For this review, take the finished solid that the model builds, in its own axes (mm). A direction names the side the tool comes from. Give positions to 0.01 mm unless a question says otherwise; leave off trailing zeros. Loops run counter-clockwise (first coordinate to the right, second up) from the corner with the lowest first, then second, coordinate; pieces in that order, holes last.
```python
from build123d import *

# Parameters (mm, degrees)
SKETCH1_R           = 6.35
BOSS_EXTRUDE1_DEPTH = 2.032
SKETCH2_R           = 4.699
BOSS_EXTRUDE2_DEPTH = 8.8646
SKETCH4_W           = 0.9906
SKETCH4_H           = 0.8509
SKETCH8_R           = 2.413
CUT_EXTRUDE2_DEPTH  = 15.24


with BuildPart() as part:
    # Sketch1 → Boss-Extrude1 (new body)
    with BuildSketch(Plane.XY):
        Circle(SKETCH1_R)
    extrude(amount=BOSS_EXTRUDE1_DEPTH)

    # Sketch2 → Boss-Extrude2 (add)
    with BuildSketch(Plane(origin=(0, 0, 0), x_dir=(-1, 0, 0), z_dir=(0, 0, -1))):
        Circle(SKETCH2_R)
    extrude(amount=BOSS_EXTRUDE2_DEPTH)

    # Sketch4 → Cut-Revolve1 (revolve, cut)
    with BuildSketch(Plane(origin=(0, 0, 0), x_dir=(0, 0, -1), z_dir=(1, 0, 0)), mode=Mode.PRIVATE) as cut_revolve1_sk:
        with Locations((7.6073, 4.27355)):
            Rectangle(SKETCH4_W, SKETCH4_H)
    revolve(cut_revolve1_sk.sketch.rotate(Axis((0, 0, 6.549062663), (0, 0, -1)), 90), axis=Axis((0, 0, 6.549062663), (0, 0, -1)), mode=Mode.SUBTRACT)

    # Sketch8 → Cut-Extrude2 (cut)
    with BuildSketch(Plane.XY.offset(2.032)):
        Circle(SKETCH8_R)
    extrude(amount=-CUT_EXTRUDE2_DEPTH, mode=Mode.SUBTRACT)


solid = part.part
```
Item 1: Tool access review of faces 5 (the cylindrical face through (-1.915, -1.468, -3.34)), 6 (the flat face through (4, 0, -7.112)), 7 (the cylindrical face through (0.61, 4.66, -3.51)): name each direction out of +Z, -Z, +X, -X, +Y, -Y from which nothing blocks a thin tool from reaching the whole face with its end or side.
Answer:
face 5: +Z, -Z
face 6: none
face 7: -Z
Item 2: Take a section at D-D on y = 0. Give the boundary of the cut face in (x, z).
Answer:
outline: (-6.35, 0) - (-4.7, 0) - (-4.7, -7.11) - (-3.85, -7.11) - (-3.85, -8.1) - (-4.7, -8.1) - (-4.7, -8.86) - (-2.41, -8.86) - (-2.41, 2.03) - (-6.35, 2.03) - close; (2.41, -8.86) - (4.7, -8.86) - (4.7, -8.1) - (3.85, -8.1) - (3.85, -7.11) - (4.7, -7.11) - (4.7, 0) - (6.35, 0) - (6.35, 2.03) - (2.41, 2.03) - close
Item 3: Take a section at C-C on z = -6.25. Give the boundary of the cut face in (x, y).
Answer:
outline: circle Ø9.4 at (0, 0); hole circle Ø4.83 at (0, 0)
Item 4: Take a section at B-B on x = 1. Give the boundary of the cut face in (y, z).
Answer:
outline: (-6.27, 0) - (-4.59, 0) - (-4.59, -7.11) - (-3.72, -7.11) - (-3.72, -8.1) - (-4.59, -8.1) - (-4.59, -8.86) - (-2.2, -8.86) - (-2.2, 2.03) - (-6.27, 2.03) - close; (2.2, -8.86) - (4.59, -8.86) - (4.59, -8.1) - (3.72, -8.1) - (3.72, -7.11) - (4.59, -7.11) - (4.59, 0) - (6.27, 0) - (6.27, 2.03) - (2.2, 2.03) - close
Item 5: Clearance check with flat-ended pins moving along their axes: pin 1 Ø6.5 at (x, y) = (1, -2) entering from -Z; pin 2 Ø1.5 at (y, z) = (-5, -5) entering from +X; pin 3 Ø2 at (y, z) = (-0.5, -3) entering from +X; pin 4 Ø1.5 at (x, z) = (-3, -4.5) entering from -Y. State where each tip first meets the part, or that it passes through.
Answer:
pin 1: stops at z = -8.86
pin 2: stops at x = 2
pin 3: stops at x = 4.7
pin 4: stops at y = -4.13
Item 6: The part is to be moulded in two halves that separate along Z. For faces 1 (the cylindrical face through (0.61, 4.66, -8.48)), 2 (the cylindrical face through (2.069, -3.245, -7.614)), 3 (the flat face through (3, 0, 2.032)), 4 (the flat face through (0, 5, 0)), say which applies: released by +Z, released by -Z, zero draft, split by the parting line, or undercut.
Answer:
face 1: zero draft
face 2: undercut
face 3: released by +Z
face 4: released by -Z
Item 7: Take a section at A-A on y = 4.5. Give the boundary of the cut face in (x, z).
Answer:
outline: (-4.48, 0) - (-1.35, 0) - (-1.35, -7.11) - (1.35, -7.11) - (1.35, 0) - (4.48, 0) - (4.48, 2.03) - (-4.48, 2.03) - close; (-1.35, -8.86) - (1.35, -8.86) - (1.35, -8.1) - (-1.35, -8.1) - close
Item 8: For L1, parallel to Z at x = 4, y = -0.25; L2, parallel to Y at x = 0, z = -4.5; L3, parallel to Z at x = 1, y = -4.75, list the stretches that pass through material, from the lowest coordinate up.
Answer:
L1: z = -8.86 to -8.1, -7.11 to 2.03
L2: y = -4.7 to -2.41, 2.41 to 4.7
L3: z = 0 to 2.03
